Check sheet for the modelled part. Datum: model origin and axes. Units: mm. Face numbers are marked on the shaded views. Give positions to 0.01 mm unless a question says otherwise; leave off trailing zeros. Loops run counter-clockwise (first coordinate to the right, second up) from the corner with the lowest first, then second, coordinate; pieces in that order, holes last. Notation, with made-up numbers: (-28, 73) - (21, 73) arc R15 cw to (21, 81) - close; hole circle Ø3 at (65, 41.5). An arc over 180 degrees is marked (long way). Use one line per item in the form item = value.
from build123d import *

# Parameters (mm, degrees)
SKETCH_W        = 20
SKETCH_H        = 20
PAD_DEPTH       = 15
SKETCH001_W     = 1.65
SKETCH001_H     = 20
POCKET_DEPTH    = 12
POCKET001_DEPTH = 20
FILLET_R        = 2
FILLET001_R     = 1


with BuildPart() as part:
    # Sketch → Pad (new body)
    with BuildSketch(Plane.XY):
        Rectangle(SKETCH_W, SKETCH_H)
    extrude(amount=PAD_DEPTH)

    # Sketch001 (on Face6 of Pad) → Pocket (cut)
    with BuildSketch(Plane.XY.offset(15)):
        Rectangle(SKETCH001_W, SKETCH001_H)
    extrude(amount=-POCKET_DEPTH, mode=Mode.SUBTRACT)

    # Sketch002 (on Face10 of Pocket) → Pocket001 (cut)
    with BuildSketch(Plane.XZ.offset(10)):
        Polygon((-10, 5), (-5, 15), (-10, 15), align=None)
    pocket001 = extrude(amount=-POCKET001_DEPTH, mode=Mode.SUBTRACT)

    # Mirrored: Pocket001 across Sketch002 V_Axis
    add(pocket001.mirror(Plane(origin=(0, -10, 0), x_dir=(0, -1, 0), z_dir=(1, 0, 0))), mode=Mode.SUBTRACT)

    # Fillet
    fillet_edges = [part.edges().sort_by_distance(p)[0] for p in [
        (5, 0, 15),
        (-5, 0, 15),
    ]]
    fillet(fillet_edges, radius=FILLET_R)

    # Fillet001
    fillet001_edges = [part.edges().sort_by_distance(p)[0] for p in [
        (-0.825, 0, 15),
        (0.825, 0, 15),
    ]]
    fillet(fillet001_edges, radius=FILLET001_R)


solid = part.part
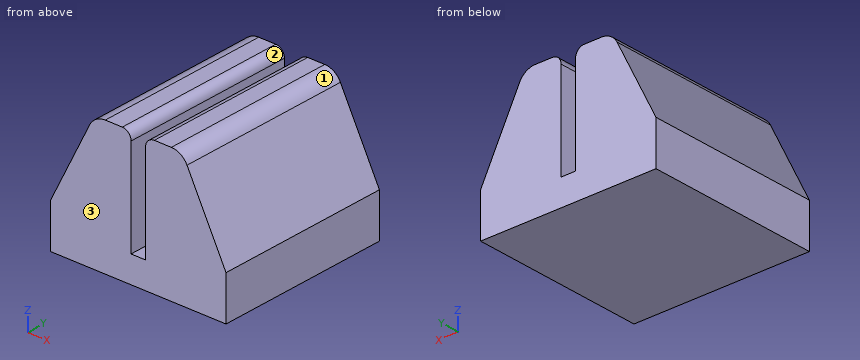
Item 1: Section check B-B on y = -3.75. Record the boundary of the cut face in (x, z) (3 decimals).
Answer block:
outline = (-10, 0) - (10, 0) - (10, 5) - (5.553, 13.894) arc R2 ccw to (3.764, 15) - (1.825, 15) arc R1 ccw to (0.825, 14) - (0.825, 3) - (-0.825, 3) - (-0.825, 14) arc R1 ccw to (-1.825, 15) - (-3.764, 15) arc R2 ccw to (-5.553, 13.894) - (-10, 5) - close
Item 2: Section check A-A on z = 8.5. Record the boundary of the cut face in (x, y) (3 decimals), then the cut area to 3 significant figures.
Answer block:
outline = (-8.25, -10) - (-0.825, -10) - (-0.825, 10) - (-8.25, 10) - close; (0.825, -10) - (8.25, -10) - (8.25, 10) - (0.825, 10) - close
area = 297 mm2
Item 3: Gauge pin test, flat ends, axial feed: P1, Ø2, axis at y = -7.5, z = 11, coming from the +X side; P2, Ø5.5, axis at y = 0.5, z = 9, coming from the -X side (3 decimals); P3, Ø1, axis at y = 5, z = 10, coming from the -X side; P4, Ø5.5, axis at y = -5, z = 7.5, coming from the +X side. Record the tip position at first contact, or that the pin passes through.
Answer block:
P1 = 7.5
P2 = -9.375
P3 = -7.75
P4 = 10
Item 4: Mould release check, pull along X, two halves, no side actions. Record for the marked faces 1, 2 and 3: released by +X, released by -X, zero draft, split by the parting line, or undercut.
Answer block:
face_1 = released by +X
face_2 = undercut
face_3 = zero draft
Item 5: Section check D-D on z = 3.75. Record the boundary of the cut face in (x, y) (3 decimals).
Answer block:
outline = (-10, -10) - (-0.825, -10) - (-0.825, 10) - (-10, 10) - close; (0.825, -10) - (10, -10) - (10, 10) - (0.825, 10) - close
Item 6: Section check C-C on x = 6. Record the boundary of the cut face in (y, z), then the cut area to 3 significant figures.
Answer block:
outline = (-10, 0) - (10, 0) - (10, 13) - (-10, 13) - close
area = 260 mm2
Item 7: Thickness scan on L1, parallel to Z at x = -0.5, y = -3.5; L2, parallel to X at y = -1, z = 11.25 (3 decimals); L3, parallel to X at y = 6.75, z = 7.75 (3 decimals). Record the ranges inside material, lowest first.
Answer block:
L1 = 0 to 3
L2 = -6.875 to -0.825, 0.825 to 6.875
L3 = -8.625 to -0.825, 0.825 to 8.625
